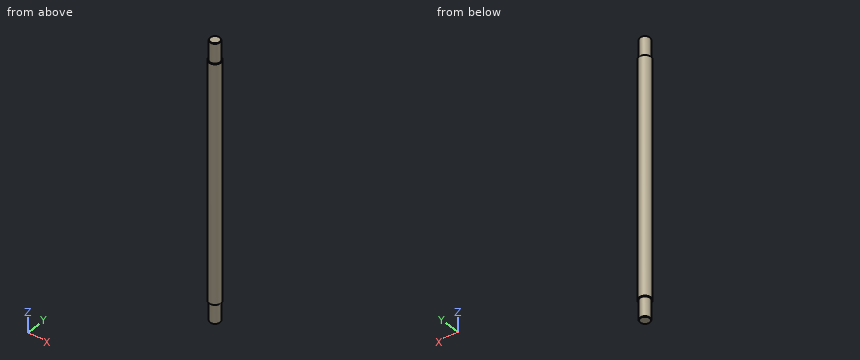
```python
from build123d import *


with BuildPart() as part:
    # Sketch1 → Revolve1 (revolve)
    with BuildSketch(Plane.XZ, mode=Mode.PRIVATE) as revolve1_sk:
        Polygon((2.3, 70), (0, 70), (0, -70), (2.3, -70), (2.5, -69.8), (2.5, -60), (3, -60), (3, 60), (2.5, 60), (2.5, 69.8), align=None)
    revolve(revolve1_sk.sketch.rotate(Axis((0, 0, 70), (0, 0, -1)), 180), axis=Axis((0, 0, 70), (0, 0, -1)))


solid = part.part
```
Can you work these out from the model? Positions are in its coordinate system, mm. Coordinates: 2 decimals unless noted, no trailing zeros. Loops run counter-clockwise (first coordinate to the right, second up) from the corner with the lowest first, then second, coordinate; pieces in that order, holes last. Notation, with made-up numbers: (3, -27.75) -> (26, -27.75) arc R25 cw to (26, -11.75) -> close; hole circle Ø1 at (26, 0.25). An arc over 180 degrees is marked (long way). Put each result on its own line as item: value. Start each with the question number.
Q1. If I drill on line 1 (Z direction, x = -0.2, y = -2.6); line 2 (Y direction, x = 1.95, z = -58.5); line 3 (Y direction, x = -0.35, z = 3.5), over which ranges is the centre line in solid material (lowest first)? Write a range as [from, to].
Q2. I want a section at C-C (z = 50). Write out the boundary of the cut face in (x, y), plus the area to 3 significant figures.
Q3. I want a section at A-A (x = 0). Write out the boundary of the cut face in (y, z), plus the area to 3 significant figures.
Taken from the geometry:
1. line 1: z = [-60, 60]
1. line 2: y = [-2.28, 2.28]
1. line 3: y = [-2.98, 2.98]
2. outline: circle Ø6 at (0, 0)
2. area: 28.3 mm2
3. outline: (-3, -60) -> (-2.5, -60) -> (-2.5, -69.8) -> (-2.3, -70) -> (2.3, -70) -> (2.5, -69.8) -> (2.5, -60) -> (3, -60) -> (3, 60) -> (2.5, 60) -> (2.5, 69.8) -> (2.3, 70) -> (-2.3, 70) -> (-2.5, 69.8) -> (-2.5, 60) -> (-3, 60) -> close
3. area: 820 mm2
